Check sheet for the modelled part. Datum: model origin and axes. Units: mm. Coordinates: 2 decimals unless noted, no trailing zeros. Loops run counter-clockwise (first coordinate to the right, second up) from the corner with the lowest first, then second, coordinate; pieces in that order, holes last. Notation, with made-up numbers: M -6.5,65 L 31.5,65 A10 cw 31.5,83 Z; hole C 85,65.25 d8. An arc over 180 degrees is marked long. Answer in a Markdown table with one row per item. Add a question column.
```python
from build123d import *

# Parameters (mm, degrees)
F0_R     = 54.402648
F0_R_2   = 43.302675
F1_DEPTH = 25.4
F2_R     = 35.004795
F2_R_2   = 27.243886
F3_DEPTH = 25.4
F4_R     = 4.445
F5_DEPTH = 25.4
F6_R     = 5.08


with BuildPart() as f1:
    # F0 (on Front) → F1 (new body)
    with BuildSketch(Plane.XZ):
        Circle(F0_R)
        Circle(F0_R_2, mode=Mode.SUBTRACT)
    extrude(amount=F1_DEPTH)



with BuildPart() as f3:
    # F2 (on Front) → F3 (new body)
    with BuildSketch(Plane.XZ):
        Circle(F2_R)
        Circle(F2_R_2, mode=Mode.SUBTRACT)
    extrude(amount=F3_DEPTH)


with BuildPart() as f1_1:
    add(f1.part)

    add(f3.part)  # F5 merges F3
    # F4 (on Front) → F5 (join)
    with BuildSketch(Plane.XZ):
        with Locations((0, 39.111675)):
            Circle(F4_R)
        with Locations((-27.65613, 27.65613)):
            Circle(F4_R)
        with Locations((-39.111675, 0)):
            Circle(F4_R)
        with Locations((-27.65613, -27.65613)):
            Circle(F4_R)
        with Locations((0, -39.111675)):
            Circle(F4_R)
        with Locations((27.65613, -27.65613)):
            Circle(F4_R)
        with Locations((39.111675, 0)):
            Circle(F4_R)
        with Locations((27.65613, 27.65613)):
            Circle(F4_R)
    extrude(amount=F5_DEPTH)

    # F6
    f6_edges = [f1_1.edges().sort_by_distance(p)[0] for p in [
        (-54.402648, -25.4, 0),
    ]]
    fillet(f6_edges, radius=F6_R)


solid = f1_1.part
```
Q1. Cross-section at B-B (z = 0). Record the cut outline in (x, y), plus the area to 3 significant figures.
Q2. Go/stop test with flat-tipped pins: pin 1 (8 mm diameter, centred on y = -4.5, z = 21.5, fed in from +X); pin 2 (5 mm diameter, centred on y = -12, z = -26, fed in from -X); pin 3 (6 mm diameter, centred on y = -14, z = 13, fed in from +X). Record where each tip stops, or that it passes through.
Q3. Mould release check, pull along Z, two halves, no side actions. Record for faces 1 (the face through (51.89, -10.02, 16.34)), 2 (the face through (21, -25.4, -21)), 3 (the face through (24.479, -12.522, -30.765)): released by +Z, released by -Z, zero draft, split by the parting line, or undercut.
Q4. Cross-section at C-C (x = 0). Record the cut outline in (y, z).
Q5. Thickness scan on L1, parallel to Z at x = 0, y = -9; L2, parallel to Z at x = -36, y = -13.5; L3, parallel to Z at x = 7, y = -12. Record the ranges inside material, lowest first.
Q6. Cross-section at A-A (y = -11). Count the separate pieces of the cut face and the enclosed holes in it, plus the area to 3 significant figures.
Answer key:
| question | item | result |
|---|---|---|
| 1 | outline | M -54.4,-20.32 A5.08 ccw -49.32,-25.4 L -27.24,-25.4 L -27.24,0 L -54.4,0 Z; M 27.24,-25.4 L 49.32,-25.4 A5.08 ccw 54.4,-20.32 L 54.4,0 L 27.24,0 Z |
| 1 | area | 1,370 mm^2 |
| 2 | pin 1 | x = 51.51 |
| 2 | pin 2 | x = -49.07 |
| 2 | pin 3 | x = 53.48 |
| 3 | face 1 | split by the parting line |
| 3 | face 2 | zero draft |
| 3 | face 3 | undercut |
| 4 | outline | M -25.4,-49.32 A5.08 ccw -20.32,-54.4 L 0,-54.4 L 0,-27.24 L -25.4,-27.24 Z; M -25.4,27.24 L 0,27.24 L 0,54.4 L -20.32,54.4 A5.08 ccw -25.4,49.32 Z |
| 5 | L1 | -54.4 to -27.24, 27.24 to 54.4 |
| 5 | L2 | -40.79 to -24.06, -3.17 to 3.17, 24.06 to 40.79 |
| 5 | L3 | -53.95 to -42.73, -34.3 to -26.33, 26.33 to 34.3, 42.73 to 53.95 |
| 6 | separate pieces | 1 |
| 6 | enclosed holes | 9 |
| 6 | area | 5,410 mm^2 |
